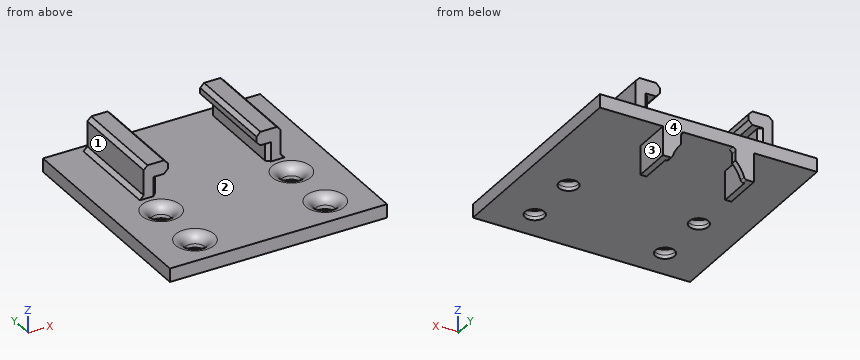
```python
from build123d import *

# Parameters (mm, degrees)
F0_W      = 57.15
F0_H      = 31.75
F0_R      = 2.54
F1_DEPTH  = 3.556
F2_W      = 57.15
F2_H      = 25.4
F3_DEPTH  = 3.556
F4_R      = 2.54
F5_W      = 3.556
F5_H      = 25.4
F6_DEPTH  = 5.08
F7_W      = 6.35
F7_H      = 25.4
F8_DEPTH  = 3.556
F9_SIZE   = 1.016
F11_DEPTH = 7.62
F12_R     = 9.8916732659
F13_DEPTH = 25.4
F14_R     = 0.8


with BuildPart() as f1:
    # F0 (on Top) → F1 (new body)
    with BuildSketch(Plane.XY):
        Rectangle(F0_W, F0_H)
        with Locations((-17.145, -7.62)):
            Circle(F0_R, mode=Mode.SUBTRACT)
        with Locations((17.145, -7.62)):
            Circle(F0_R, mode=Mode.SUBTRACT)
        with Locations((-17.145, 7.62)):
            Circle(F0_R, mode=Mode.SUBTRACT)
        with Locations((17.145, 7.62)):
            Circle(F0_R, mode=Mode.SUBTRACT)
    extrude(amount=F1_DEPTH)

    # F2 (on Top) → F3 (join)
    with BuildSketch(Plane.XY):
        with Locations((0, 28.575)):
            Rectangle(F2_W, F2_H)
    extrude(amount=F3_DEPTH)

    # F4
    f4_edges = [f1.edges().sort_by_distance(p)[0] for p in [
        (-19.685, 7.62, 3.556),
        (14.605, 7.62, 3.556),
        (14.605, -7.62, 3.556),
        (-19.685, -7.62, 3.556),
    ]]
    fillet(f4_edges, radius=F4_R)

    # F5 (on face) → F6 (join)
    with BuildSketch(Plane.XY.offset(3.556)):
        with Locations((-16.256, 26.67)):
            Rectangle(F5_W, F5_H)
        with Locations((16.256, 26.67)):
            Rectangle(F5_W, F5_H)
    extrude(amount=F6_DEPTH)

    # F7 (on face) → F8 (join)
    with BuildSketch(Plane.XY.offset(8.636)):
        with Locations((-14.859, 26.67)):
            Rectangle(F7_W, F7_H)
        with Locations((14.859, 26.67)):
            Rectangle(F7_W, F7_H)
    extrude(amount=F8_DEPTH)

    # F9
    f9_edges = [f1.edges().sort_by_distance(p)[0] for p in [
        (-11.684, 26.67, 12.192),
        (-11.684, 26.67, 8.636),
        (11.684, 26.67, 12.192),
        (11.684, 26.67, 8.636),
        (18.034, 26.67, 12.192),
        (-18.034, 26.67, 12.192),
        (18.034, 26.67, 3.556),
        (-18.034, 26.67, 3.556),
        (14.478, 39.37, 6.096),
        (-14.478, 39.37, 6.096),
        (-14.478, 13.97, 6.096),
        (14.478, 13.97, 6.096),
    ]]
    chamfer(f9_edges, length=F9_SIZE)

    # F10 (on face) → F11 (join)
    with BuildSketch(Plane(origin=(0, 0, 0), x_dir=(1, 0, 0), z_dir=(0, 0, -1))):
        Polygon((-11.96, -41.275), (-7.16, -41.275), (-7.16, -39.675), (-10.36, -39.675), (-10.36, -31.115), (-11.96, -31.115), align=None)
        Polygon((10.36, -31.115), (10.36, -39.675), (7.16, -39.675), (7.16, -41.275), (11.96, -41.275), (11.96, -31.115), align=None)
    extrude(amount=F11_DEPTH)

    # F12 (on face) → F13 (cut)
    with BuildSketch(Plane(origin=(0, 41.275, 0), x_dir=(-1, 0, 0), z_dir=(0, 1, 0))):
        with Locations((0, -10.16)):
            Circle(F12_R)
    extrude(amount=-F13_DEPTH, mode=Mode.SUBTRACT)

    # F14
    f14_edges = [f1.edges().sort_by_distance(p)[0] for p in [
        (9.56, 40.475, -7.62),
        (-9.56, 40.475, -7.62),
        (-7.16, 40.475, 0),
        (7.16, 40.475, 0),
    ]]
    fillet(f14_edges, radius=F14_R)


solid = f1.part
```
Check sheet for the modelled part. Datum: model origin and axes. Units: mm. Face numbers are marked on the shaded views. Give positions to 0.01 mm unless a question says otherwise; leave off trailing zeros. Order: outer loops, then holes, each group sorted by start corner. A loop starts at its lowest first (then second) coordinate and runs counter-clockwise, first axis right, second up. Notation, with made-up numbers: (-31.5, -12) -> (-14.5, -12) arc R20 ccw to (-14.5, 0) -> close; hole circle Ø2 at (22.25, 67). An arc over 180 degrees is marked (long way). Return JSON: item names as keys, results as strings.
1. Go/stop test with flat-tipped pins: P1, Ø2, axis at y = 30.5, z = -4, coming from the +X side; P2, Ø1.3, axis at x = 11, z = -5, coming from the -Y side (3 decimals); P3, Ø3, axis at x = -13.5, y = 28, coming from the -Z side; P4, Ø5, axis at x = -5.5, z = 8, coming from the +Y side. Record where each tip stops, or that it passes through.
From the geometry:
{"P1": "x = 11.96", "P2": "y = 31.115", "P3": "z = 0", "P4": "through"}
2. Mould release check, pull along X, two halves, no side actions. Record for the marked faces 1, 2, 3 and 4: +X half, -X half, draft (parallel to the pull), parting line (faces both ways), or undercut.
From the geometry:
{"face 1": "-X half", "face 2": "undercut", "face 3": "+X half", "face 4": "draft"}
3. Cross-section at B-B, the plane y = 7.62. Record the cut outline in (x, z) (3 decimals), plus the area to 3 significant figures.
From the geometry:
{"outline": "(-28.575, 0) -> (-19.685, 0) -> (-19.685, 1.016) arc R2.54 ccw to (-22.225, 3.556) -> (-28.575, 3.556) -> close; (-14.605, 0) -> (14.605, 0) -> (14.605, 1.016) arc R2.54 ccw to (12.065, 3.556) -> (-12.065, 3.556) arc R2.54 ccw to (-14.605, 1.016) -> close; (19.685, 0) -> (28.575, 0) -> (28.575, 3.556) -> (22.225, 3.556) arc R2.54 ccw to (19.685, 1.016) -> close", "area": "162 mm^2"}
4. Cross-section at A-A, the plane z = 6.25. Record the cut outline in (x, y), plus the area to 3 significant figures.
From the geometry:
{"outline": "(-18.03, 13.97) -> (-15.49, 13.97) -> (-14.48, 14.99) -> (-14.48, 38.35) -> (-15.49, 39.37) -> (-18.03, 39.37) -> close; (14.48, 14.99) -> (15.49, 13.97) -> (18.03, 13.97) -> (18.03, 39.37) -> (15.49, 39.37) -> (14.48, 38.35) -> close", "area": "179 mm^2"}
5. Material ranges on probe 1 along X at (y, z) = (32, 8.25); probe 2 along Y at (x, z) = (-10.5, -6.75) (3 decimals); probe 3 along Z at (x, y) = (-10, 1.5), recorded low to high. Write a range as [from, to].
From the geometry:
{"probe 1": "[-18.03, -14.48], [14.48, 18.03]", "probe 2": "[31.115, 41.275]", "probe 3": "[0, 3.56]"}
6. Cross-section at D-D, the plane x = 0. Record the cut outline in (y, z) (3 decimals), plus the area to 3 significant figures.
From the geometry:
{"outline": "(-15.875, 0) -> (41.275, 0) -> (41.275, 3.556) -> (-15.875, 3.556) -> close", "area": "203 mm^2"}
